```python
from build123d import *

# Parameters (mm, degrees)
BOSS_EXTRUDE1_DEPTH = 1.524


with BuildPart() as part:
    # Sketch1 → Boss-Extrude1 (new body)
    with BuildSketch(Plane.XY):
        with BuildLine():
            Line((-4.3376529, 0), (-4.3376529, 1.524))
            Line((-4.3376529, 1.524), (-5.8616529, 1.524))
            Line((-5.8616529, 1.524), (-5.8616529, 0))
            Line((-5.8616529, 0), (-6.478290939, 0))
            Line((-6.478290939, 0), (-6.478290939, -0.743115039))
            ThreePointArc((-6.478290939, -0.743115039), (-6.511193249, -0.964611222), (-6.60705881, -1.166979488))
            ThreePointArc((-6.60705881, -1.166979488), (-15.054242265, -8.616097958), (-26.078104852, -10.922334716))
            ThreePointArc((-26.078104852, -10.922334716), (-23.165548821, -11.565461887), (-20.18747251, -11.731764839))
            Line((-20.18747251, -11.731764839), (-19.700670178, -12.287185002))
            Line((-19.700670178, -12.287185002), (-19.547051581, -11.704642596))
            ThreePointArc((-19.547051581, -11.704642596), (-17.624782342, -11.488416043), (-15.735636356, -11.072482882))
            Line((-15.735636356, -11.072482882), (-15.043782744, -11.466191113))
            Line((-15.043782744, -11.466191113), (-15.154372523, -10.901903689))
            ThreePointArc((-15.154372523, -10.901903689), (-13.71444875, -10.38734424), (-12.321981989, -9.755530806))
            Line((-12.321981989, -9.755530806), (-11.499632126, -10.334098846))
            Line((-11.499632126, -10.334098846), (-11.840203527, -9.503461421))
            ThreePointArc((-11.840203527, -9.503461421), (-10.331263681, -8.589737909), (-8.916295851, -7.536335727))
            Line((-8.916295851, -7.536335727), (-7.998857494, -8.049594043))
            Line((-7.998857494, -8.049594043), (-8.574085726, -7.248219572))
            ThreePointArc((-8.574085726, -7.248219572), (-7.68975334, -6.433548021), (-6.860257429, -5.563105582))
            Line((-6.860257429, -5.563105582), (-5.8616529, -5.685853343))
            Line((-5.8616529, -5.685853343), (-6.578924281, -5.240527193))
            ThreePointArc((-6.578924281, -5.240527193), (-5.71334828, -4.14305213), (-4.933175939, -2.983308863))
            Line((-4.933175939, -2.983308863), (-3.82490487, -2.830476181))
            Line((-3.82490487, -2.830476181), (-4.739829013, -2.663849113))
            ThreePointArc((-4.739829013, -2.663849113), (-4.258864728, -1.798680626), (-3.82490487, -0.909005407))
            ThreePointArc((-3.82490487, -0.909005407), (-3.801959849, -0.852730225), (-3.783572445, -0.794805504))
            Line((-3.783572445, -0.794805504), (-3.565751855, 0))
            Line((-3.565751855, 0), (-4.3376529, 0))
        make_face()
    extrude(amount=BOSS_EXTRUDE1_DEPTH)


solid = part.part
```
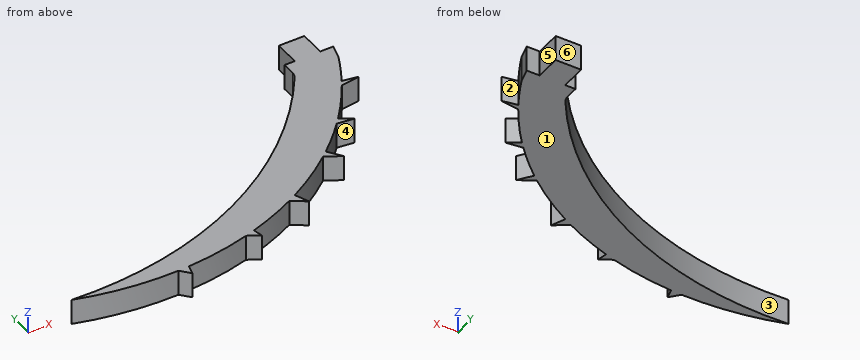
Geometry check sheet. Reference: the model listing, model coordinates, mm. Face numbers are marked on the shaded views. A direction names the side the tool comes from. Give positions to 0.01 mm unless a question says otherwise; leave off trailing zeros. Loops run counter-clockwise (first coordinate to the right, second up) from the corner with the lowest first, then second, coordinate; pieces in that order, holes last. Notation, with made-up numbers: M 33,66 L 65,66 A9 cw 65,72 Z; hole C -19,48 d6. An arc over 180 degrees is marked long. Write item = value, one per line. Start each with the question number.
1. Section check C-C, the plane x = -16.25. Enter the section's corners in (y, z), plus the area to 3 significant figures.
2. Go/stop test with flat-tipped pins: P1, Ø8, axis at x = -15.5, y = -10.5, coming from the -Z side; P2, Ø0.5, axis at y = 1, z = 0.5, coming from the -X side; P3, Ø0.8, axis at y = 0.5, z = 1, coming from the +X side. Record where each tip stops, or that it passes through.
3. Draft check along Y on the marked faces 1, 2 and 3. Enter one of: +Y half, -Y half, draft (parallel to the pull), parting line (faces both ways), or undercut.
4. Tool access check on the marked faces 4, 5 and 6. Record the directions out of +Z, -Z, +X, -X, +Y, -Y that give a thin tool (end or side, any length) a straight path to the whole face; none if there is none.
5. Section check D-D, the plane y = -6. Enter the section's corners in (x, z).
6. Thickness scan on probe 1 along Y at (x, z) = (-10.5, 0.7); probe 2 along Y at (x, z) = (-14.25, 1.3); probe 3 along X at (y, z) = (-5.5, 0.7). Record the ranges inside material, lowest first.
7. Section check A-A, the plane y = -7.75. Enter the section's corners in (x, z), plus the area to 3 significant figures.
Values follow:
q1.outline = M -11.21,0 L -9.17,0 L -9.17,1.52 L -11.21,1.52 Z
q1.area = 3.10 mm^2
q2.P1 = 0
q2.P2 = -5.86
q2.P3 = -4.34
q3.face_1 = draft
q3.face_2 = undercut
q3.face_3 = +Y half
q4.face_4 = +Z, -Z, -Y
q4.face_5 = +Z, -Z, +X, +Y
q4.face_6 = +Z, -Z, +X, -X, +Y
q5.outline = M -11.01,0 L -7.26,0 L -7.26,1.52 L -11.01,1.52 Z
q6.probe_1 = -8.7 to -5.57
q6.probe_2 = -10.59 to -8.19
q6.probe_3 = -10.42 to -6.16
q7.outline = M -13.49,0 L -9.18,0 L -9.18,1.52 L -13.49,1.52 Z; M -8.53,0 L -8.21,0 L -8.21,1.52 L -8.53,1.52 Z
q7.area = 7.05 mm^2
